```python
from build123d import *

# Parameters (mm, degrees)
FILLET1_R = 0.25


with BuildPart() as part:
    # Sketch1 → Revolve1 (revolve)
    with BuildSketch(Plane.XY):
        Polygon((4.75, 10), (9.75, 10), (12.5, 2.25), (12.5, 0), (4.75, 0), align=None)
    revolve(axis=Axis((0, 0, 0), (0, 1, 0)))

    # Fillet1
    fillet1_edges = [part.edges().sort_by_distance(p)[0] for p in [
        (-4.75, 0, 0),
        (-12.5, 0, 0),
        (-12.5, 2.25, 0),
        (-9.75, 10, 0),
        (-4.75, 10, 0),
    ]]
    fillet(fillet1_edges, radius=FILLET1_R)


solid = part.part
```
Here's how the part is built. I have some questions about the finished solid (model axes, mm). Coordinates: 2 decimals unless noted, no trailing zeros. Write each loop counter-clockwise with the first axis right and the second up, starting at its lowest first coordinate (ties: lowest second). Pieces come first, ordered by that corner, then holes. Notation, with made-up numbers: (59.5, -0.5) -> (73.5, -0.5) arc R26 cw to (73.5, 27.5) -> close; hole circle Ø3 at (43.5, 47). An arc over 180 degrees is marked (long way). Use a Markdown table: item, result. Add a question column.
(1) If we section it at A-A, the plane y = 0.75: Write out the boundary of the cut face in (x, z).
(2) I'm going to push flat-ended pins straight in: P1, Ø2, axis at x = -1, y = 7.5, coming from the +Z side; P2, Ø2, axis at y = 8, z = -8.5, coming from the -X side; P3, Ø2, axis at x = -3, y = 7, coming from the -Z side; P4, Ø8.5, axis at x = 0, z = 0, coming from the +Y side. Where does each tip first touch, or does it pass through?
(3) We'd pull the mould along Z, two halves only. Please class faces 1 (the conical face through (-2.16, 9.36, 9.74)), 2 (the cylindrical face through (2.192, 5.066, 4.214)), 3 (the flat face through (5.3, 0, -0.2)): +Z half, -Z half, draft (parallel to the pull), parting line (faces both ways), or undercut.
(4) Please list where these lines run through material, in increasing order: line 1 (Z direction, x = 1, y = 7.5); line 2 (Z direction, x = 3, y = 3.25); line 3 (X direction, y = 2.5, z = 0).
(5) If we section it at B-B, the plane y = 6: Write out the boundary of the cut face in (x, z), and give its area (3 significant figures).
Outcome:
| question | item | result |
|---|---|---|
| 1 | outline | circle Ø25 at (0, 0); hole circle Ø9.5 at (0, 0) |
| 2 | P1 | stops at z = 10.96 |
| 2 | P2 | stops at x = -7.41 |
| 2 | P3 | stops at z = -10.84 |
| 2 | P4 | passes through |
| 3 | face 1 | parting line |
| 3 | face 2 | undercut |
| 3 | face 3 | draft |
| 4 | line 1 | z = -10.59 to -4.64, 4.64 to 10.59 |
| 4 | line 2 | z = -11.77 to -3.68, 3.68 to 11.77 |
| 4 | line 3 | x = -12.41 to -4.75, 4.75 to 12.41 |
| 5 | outline | circle Ø22.34 at (0, 0); hole circle Ø9.5 at (0, 0) |
| 5 | area | 321 mm^2 |
